Input: part model. Units: mm. Frame: model coordinates. A direction names the side the tool comes from. Round coordinates to 2 decimals unless told otherwise and drop trailing zeros. Loops run counter-clockwise (first coordinate to the right, second up) from the corner with the lowest first, then second, coordinate; pieces in that order, holes last. Notation, with made-up numbers: M 41.25,41.5 L 77.25,41.5 A18 ccw 77.25,61.5 Z; hole C -32.5,3 d10. An arc over 180 degrees is marked long. Return JSON: item names as keys, results as strings. Group by question number.
1) Contact query for flat-ended pins moving along their axis: P1, Ø4, axis at x = -44, y = 19.5, coming from the -Z side; P2, Ø5.5, axis at x = -69.5, z = 31.5, coming from the +Y side; P3, Ø6, axis at x = -58, z = 8, coming from the -Y side; P4, Ø3, axis at y = -5.5, z = 40.5, coming from the -X side. Output: stop coordinate, or through.
2) Material intervals for line 1 (X direction, y = 10, z = 33.5); line 2 (Y direction, x = -71.5, z = 23); line 3 (Y direction, x = -26, z = 39), sorted ascending. Write a range as from..to.
3) Mould query, pull axis X, two halves, no side actions, for faces 4 (the face through (-39.641, -2.815, 22.185)), 5 (the face through (-53.486, 28.163, 22.185)), 6 (the face through (-29, 16, 0)). Classes: +X half, -X half, draft (parallel to the pull), parting line (faces both ways), or undercut.
4) Section C-C (z = 34). Output: boundary loops of the cut face in (x, y), plus the area to 3 significant figures.
5) Section A-A (x = -60). Output: boundary loops of the cut face in (y, z), plus the area to 3 significant figures.
6) Section B-B (y = 18). Output: boundary loops of the cut face in (x, z), plus the area to 3 significant figures.
7) Section D-D (y = -3). Output: boundary loops of the cut face in (x, z), plus the area to 3 significant figures.
8) Access query for faces 1 (the face through (-58, -1.634, 22)), 2 (the face through (-72.657, 10.264, 22.185)), 3 (the face through (-69, 30.366, 22)). Directions: +Z, -Z, +X, -X, +Y, -Y. A direction counts if a zero-diameter tool reaches every point of the face in a straight line with its end or side. Return the directions, or none.
from build123d import *

# Parameters (mm, degrees)
SKETCH1_R           = 7
BOSS_EXTRUDE1_DEPTH = 45


with BuildPart() as part:
    # Sketch1 → Boss-Extrude1 (new body)
    with BuildSketch(Plane.XY):
        with BuildLine():
            ThreePointArc((-42.867935385, -1.633500031), (-39.602699604, -2.846913799), (-37.922296644, -5.898205914))
            ThreePointArc((-37.922296644, -5.898205914), (-35.585466441, -13.749172092), (-31.146494244, -20.633500031))
            Line((-31.146494244, -20.633500031), (-24.980449087, -20.633500031))
            Line((-24.980449087, -20.633500031), (4.019550913, 14.366499969))
            Line((4.019550913, 14.366499969), (4.019550913, 33.366499969))
            Line((4.019550913, 33.366499969), (-0.980449087, 38.366499969))
            Line((-0.980449087, 38.366499969), (-24.980449087, 38.366499969))
            ThreePointArc((-24.980449087, 38.366499969), (-30.471993331, 28.634090038), (-41.337061073, 26.021205766))
            Line((-41.337061073, 26.021205766), (-65.980449087, 30.366499969))
            Line((-65.980449087, 30.366499969), (-72.980449087, 30.366499969))
            Line((-72.980449087, 30.366499969), (-79.980449087, 23.366499969))
            Line((-79.980449087, 23.366499969), (-79.980449087, 5.366499969))
            Line((-79.980449087, 5.366499969), (-72.980449087, -1.633500031))
            Line((-72.980449087, -1.633500031), (-42.867935385, -1.633500031))
        make_face()
        with Locations(Location((-65.980449087, 12.366499969, 0), (0, 0, 180))):
            Circle(SKETCH1_R, mode=Mode.SUBTRACT)
    extrude(amount=BOSS_EXTRUDE1_DEPTH)


solid = part.part
Returned:
{
 "1": {"P1": "stops at z = 0", "P2": "stops at y = 30.37", "P3": "stops at y = -1.63", "P4": "stops at x = -38.62"},
 "2": {"line 1": "x = -79.98..-72.57, -59.39..0.4", "line 2": "y = -1.63..8.06, 16.67..30.37", "line 3": "y = -20.63..34.38"},
 "3": {"face 4": "-X half", "face 5": "undercut", "face 6": "draft"},
 "4": {"outline": "M -79.98,5.37 L -72.98,-1.63 L -42.87,-1.63 A5 cw -37.92,-5.9 A29 ccw -31.15,-20.63 L -24.98,-20.63 L 4.02,14.37 L 4.02,33.37 L -0.98,38.37 L -24.98,38.37 A14 cw -41.34,26.02 L -65.98,30.37 L -72.98,30.37 L -79.98,23.37 Z; hole C -65.98,12.37 d14", "area": "2,870 mm^2"},
 "5": {"outline": "M -1.63,0 L 8.73,0 L 8.73,45 L -1.63,45 Z; M 16,0 L 29.31,0 L 29.31,45 L 16,45 Z", "area": "1,070 mm^2"},
 "6": {"outline": "M -79.98,0 L -70.14,0 L -70.14,45 L -79.98,45 Z; M -61.83,0 L 4.02,0 L 4.02,45 L -61.83,45 Z", "area": "3,410 mm^2"},
 "7": {"outline": "M -39.43,0 L -10.37,0 L -10.37,45 L -39.43,45 Z", "area": "1,310 mm^2"},
 "8": {"face 1": "+Z, -Z, -X, -Y", "face 2": "+Z, -Z", "face 3": "+Z, -Z, -X, +Y"}
}
